Geometry: final body of the model. Coordinates: model frame, mm. A direction names the side the tool comes from. Give positions to 0.01 mm unless a question says otherwise; leave off trailing zeros. Write each loop counter-clockwise with the first axis right and the second up, starting at its lowest first coordinate (ties: lowest second). Pieces come first, ordered by that corner, then holes. Notation, with made-up numbers: M 25,56.25 L 78,56.25 A17 ccw 78,67.25 Z; hole C 7.25,19.25 d1. An arc over 180 degrees is marked long. One line per question, with ' | ' between items.
from build123d import *

# Parameters (mm, degrees)
EXTRUDE_1_DEPTH           = 50
HOLE_WIZARD_6_0_6_1_DEPTH = 1
PATTERN_LINEAR_1_COUNT    = 3
PATTERN_LINEAR_1_PITCH    = 25
MIRROR_1_COPY_1_DEPTH     = 1
MIRROR_1_COPY_2_DEPTH     = 1
MIRROR_1_COPY_3_DEPTH     = 1


# Read off the part's stored shape, not the designer's step: Диаметр отверстия Ø6.0 (6)1
with BuildPart() as part:
    # Эскиз1 → Вытянуть-Тонкостенный1 (new, symmetric)
    with BuildSketch(Plane(origin=(0, 0, 0), x_dir=(0, 0, -1), z_dir=(1, 0, 0))):
        with BuildLine():
            Line((-6.5, -17.5), (-6.5, -14))
            ThreePointArc((-6.5, -14), (-6.353553391, -13.646446609), (-6, -13.5))
            Line((-6, -13.5), (-1.5, -13.5))
            ThreePointArc((-1.5, -13.5), (-0.439339828, -13.060660172), (0, -12))
            Line((0, -12), (0, 12))
            ThreePointArc((0, 12), (-0.439339828, 13.060660172), (-1.5, 13.5))
            Line((-1.5, 13.5), (-6, 13.5))
            ThreePointArc((-6, 13.5), (-6.353553391, 13.646446609), (-6.5, 14))
            Line((-6.5, 14), (-6.5, 17.5))
            Line((-6.5, 17.5), (-7.5, 17.5))
            Line((-7.5, 17.5), (-7.5, 14))
            ThreePointArc((-7.5, 14), (-7.060660172, 12.939339828), (-6, 12.5))
            Line((-6, 12.5), (-1.5, 12.5))
            ThreePointArc((-1.5, 12.5), (-1.146446609, 12.353553391), (-1, 12))
            Line((-1, 12), (-1, -12))
            ThreePointArc((-1, -12), (-1.146446609, -12.353553391), (-1.5, -12.5))
            Line((-1.5, -12.5), (-6, -12.5))
            ThreePointArc((-6, -12.5), (-7.060660172, -12.939339828), (-7.5, -14))
            Line((-7.5, -14), (-7.5, -17.5))
            Line((-7.5, -17.5), (-6.5, -17.5))
        make_face()
    extrude(amount=EXTRUDE_1_DEPTH, both=True)

    # Диаметр отверстия Ø6.0 (6)1 outline → Диаметр отверстия Ø6.0 (6)1 (cut)
    with BuildSketch(Plane.XY):
        with BuildLine():
            Line((-6, -3), (6, -3))
            ThreePointArc((6, -3), (9, 0), (6, 3))
            Line((6, 3), (-6, 3))
            ThreePointArc((-6, 3), (-9, 0), (-6, -3))
        make_face()
    hole_wizard_6_0_6_1 = extrude(amount=HOLE_WIZARD_6_0_6_1_DEPTH, mode=Mode.SUBTRACT)

    # Линейный массив1: Диаметр отверстия Ø6.0 (6)1 ×3
    with Locations(*[(i * PATTERN_LINEAR_1_PITCH, 0, 0) for i in range(1, PATTERN_LINEAR_1_COUNT)]):
        add(hole_wizard_6_0_6_1, mode=Mode.SUBTRACT)

    # Зеркальное отражение1 copy 1 sketch → Зеркальное отражение1 copy 1 (cut)
    with BuildSketch(Plane(origin=(-25, 0, 0), x_dir=(-1, 0, 0), z_dir=(0, 0, 1))):
        with BuildLine():
            Line((-6, 3), (6, 3))
            ThreePointArc((6, 3), (9, 0), (6, -3))
            Line((6, -3), (-6, -3))
            ThreePointArc((-6, -3), (-9, 0), (-6, 3))
        make_face()
    extrude(amount=MIRROR_1_COPY_1_DEPTH, mode=Mode.SUBTRACT)

    # Зеркальное отражение1 copy 2 sketch → Зеркальное отражение1 copy 2 (cut)
    with BuildSketch(Plane(origin=(-50, 0, 0), x_dir=(-1, 0, 0), z_dir=(0, 0, 1))):
        with BuildLine():
            Line((-6, 3), (6, 3))
            ThreePointArc((6, 3), (9, 0), (6, -3))
            Line((6, -3), (-6, -3))
            ThreePointArc((-6, -3), (-9, 0), (-6, 3))
        make_face()
    extrude(amount=MIRROR_1_COPY_2_DEPTH, mode=Mode.SUBTRACT)

    # Зеркальное отражение1 copy 3 sketch → Зеркальное отражение1 copy 3 (cut)
    with BuildSketch(Plane(origin=(0, 0, 0), x_dir=(-1, 0, 0), z_dir=(0, 0, 1))):
        with BuildLine():
            Line((-6, 3), (6, 3))
            ThreePointArc((6, 3), (9, 0), (6, -3))
            Line((6, -3), (-6, -3))
            ThreePointArc((-6, -3), (-9, 0), (-6, 3))
        make_face()
    extrude(amount=MIRROR_1_COPY_3_DEPTH, mode=Mode.SUBTRACT)


solid = part.part
(1) Cut plane B-B, the plane x = -38. Return loops of the section in (y, z).
Working result:
outline: M -17.5,6.5 L -14,6.5 A0.5 cw -13.5,6 L -13.5,1.5 A1.5 ccw -12,0 L 12,0 A1.5 ccw 13.5,1.5 L 13.5,6 A0.5 cw 14,6.5 L 17.5,6.5 L 17.5,7.5 L 14,7.5 A1.5 ccw 12.5,6 L 12.5,1.5 A0.5 cw 12,1 L -12,1 A0.5 cw -12.5,1.5 L -12.5,6 A1.5 ccw -14,7.5 L -17.5,7.5 Z
(2) Cut plane A-A, the plane x = 30. Return loops of the section in (y, z).
Working result:
outline: M -17.5,6.5 L -14,6.5 A0.5 cw -13.5,6 L -13.5,1.5 A1.5 ccw -12,0 L -3,0 L -3,1 L -12,1 A0.5 cw -12.5,1.5 L -12.5,6 A1.5 ccw -14,7.5 L -17.5,7.5 Z; M 3,0 L 12,0 A1.5 ccw 13.5,1.5 L 13.5,6 A0.5 cw 14,6.5 L 17.5,6.5 L 17.5,7.5 L 14,7.5 A1.5 ccw 12.5,6 L 12.5,1.5 A0.5 cw 12,1 L 3,1 Z
(3) Material intervals for L1, parallel to Y at x = 19, z = 3.5; L2, parallel to Z at x = -4, y = 15; L3, parallel to Z at x = 22.5, y = -7.5, sorted ascending. Write a range as [from, to].
Working result:
L1: y = [-13.5, -12.5], [12.5, 13.5] | L2: z = [6.5, 7.5] | L3: z = [0, 1]
(4) First-contact query: P1, Ø1.3, axis at x = -7.5, z = 3, coming from the -Y side; P2, Ø1, axis at y = 0.5, z = 1, coming from the +X side; P3, Ø0.8, axis at x = -2, z = 0.5, coming from the -Y side. Flat tips, straight axial feed; report the tip coordinate or a pass-through.
Working result:
P1: stops at y = -13.5 | P2: stops at x = 41.17 | P3: stops at y = -13.37
(5) Set-up query: faces 5 (the face through (1, 16, 6.5)), 6 (the face through (1, 6, 1)), 7 (the face through (1, -16, 6.5)). Return all of +Z, -Z, +X, -X, +Y, -Y with unobstructed straight access to the full face (end or side cutting, diameter ignored); none if empty.
Working result:
face 5: -Z, +X, -X, +Y | face 6: +Z, +X, -X | face 7: -Z, +X, -X, -Y
(6) Cut plane C-C, the plane y = -4. Return loops of the section in (x, z).
Working result:
outline: M -50,0 L 50,0 L 50,1 L -50,1 Z
(7) Draft query along Y for faces 1 (the face through (-34, -0.1, 0.5)), 2 (the face through (34, -0.1, 0.5)), 3 (the face through (50, 10.8, 0.7)), 4 (the face through (1, 13.5, 4)). Return one class per face: released by +Y, released by -Y, zero draft, split by the parting line, or undercut.
Working result:
face 1: undercut | face 2: undercut | face 3: zero draft | face 4: released by +Y
